from build123d import *

# Parameters (mm, degrees)
SKETCH1_R           = 5
BOSS_EXTRUDE1_DEPTH = 8
SKETCH2_R           = 17.5
BOSS_EXTRUDE2_DEPTH = 5
BOSS_EXTRUDE3_START = 7.75
SKETCH3_R           = 17.5
SKETCH3_R_2         = 13.5
BOSS_EXTRUDE3_DEPTH = 7.75
SKETCH4_R           = 6
BOSS_EXTRUDE4_DEPTH = 58.4
SKETCH7_R           = 7.998050104
SKETCH7_R_2         = 4
CUT_EXTRUDE1_DEPTH  = 30
SKETCH8_R           = 8
SKETCH8_R_2         = 6
BOSS_EXTRUDE6_DEPTH = 9
BOSS_EXTRUDE7_START = 5
BOSS_EXTRUDE7_DEPTH = 5


with BuildPart() as part:
    # Sketch1 → Boss-Extrude1 (new body)
    with BuildSketch(Plane(origin=(0, 0, 0), x_dir=(1, 0, 0), z_dir=(0, 1, 0))):
        with Locations(Location((0, 0, 0), (0, 0, 270))):
            Circle(SKETCH1_R)
    extrude(amount=-BOSS_EXTRUDE1_DEPTH)

    # Sketch2 → Boss-Extrude2 (add)
    with BuildSketch(Plane(origin=(0, 0, 0), x_dir=(1, 0, 0), z_dir=(0, 1, 0))):
        with Locations(Location((0, 0, 0), (0, 0, 270))):
            Circle(SKETCH2_R)
    extrude(amount=BOSS_EXTRUDE2_DEPTH)

    # Sketch3 → Boss-Extrude3 (add)
    with BuildSketch(Plane.XZ.offset(BOSS_EXTRUDE3_START)):
        with Locations(Location((0, 0, 0), (0, 0, 270))):
            Circle(SKETCH3_R)
        with Locations(Location((0, 0, 0), (0, 0, 270))):
            Circle(SKETCH3_R_2, mode=Mode.SUBTRACT)
    extrude(amount=-BOSS_EXTRUDE3_DEPTH)

    # Sketch4 → Boss-Extrude4 (add)
    with BuildSketch(Plane(origin=(0, 5, 0), x_dir=(1, 0, 0), z_dir=(0, 1, 0))):
        with Locations(Location((0, 0, 0), (0, 0, 270))):
            Circle(SKETCH4_R)
    extrude(amount=BOSS_EXTRUDE4_DEPTH)

    # Sketch7 → Cut-Extrude1 (cut)
    with BuildSketch(Plane(origin=(0, 63.4, 0), x_dir=(1, 0, 0), z_dir=(0, 1, 0))):
        Circle(SKETCH7_R)
        with Locations(Location((0, 0, 0), (0, 0, 270))):
            Circle(SKETCH7_R_2, mode=Mode.SUBTRACT)
    extrude(amount=-CUT_EXTRUDE1_DEPTH, mode=Mode.SUBTRACT)

    # Sketch8 → Boss-Extrude6 (add)
    with BuildSketch(Plane(origin=(0, 5, 0), x_dir=(1, 0, 0), z_dir=(0, 1, 0))):
        with Locations(Location((0, 0, 0), (0, 0, 270))):
            Circle(SKETCH8_R)
        with Locations(Location((0, 0, 0), (0, 0, 270))):
            Circle(SKETCH8_R_2, mode=Mode.SUBTRACT)
    extrude(amount=BOSS_EXTRUDE6_DEPTH)

    # Sketch10 → Boss-Extrude7 (add)
    with BuildSketch(Plane(origin=(0, 63.4, 0), x_dir=(1, 0, 0), z_dir=(0, 1, 0)).offset(BOSS_EXTRUDE7_START)):
        with BuildLine():
            Line((-3.25, 2.331844763), (-3.25, -2.331844763))
            ThreePointArc((-3.25, -2.331844763), (-2.828427125, -2.828427125), (-2.331844763, -3.25))
            Line((-2.331844763, -3.25), (2.331844763, -3.25))
            ThreePointArc((2.331844763, -3.25), (2.828427125, -2.828427125), (3.25, -2.331844763))
            Line((3.25, -2.331844763), (3.25, 2.331844763))
            ThreePointArc((3.25, 2.331844763), (2.828427125, 2.828427125), (2.331844763, 3.25))
            Line((2.331844763, 3.25), (-2.331844763, 3.25))
            ThreePointArc((-2.331844763, 3.25), (-2.828427125, 2.828427125), (-3.25, 2.331844763))
        make_face()
    extrude(amount=-BOSS_EXTRUDE7_DEPTH)


solid = part.part
Could you check a few things on this model? Use its own coordinates, in mm. A direction names the side the tool comes from. Give positions to 0.01 mm unless a question says otherwise; leave off trailing zeros. Order: outer loops, then holes, each group sorted by start corner. A loop starts at its lowest first (then second) coordinate and runs counter-clockwise, first axis right, second up. Notation, with made-up numbers: (-28, 70) - (29, 70) arc R19 cw to (29, 102) - close; hole circle Ø3 at (-6.75, 37.25). An arc over 180 degrees is marked (long way). One line per item, written item: value. Start each with the question number.
1. Imagine slicing it at B-B on z = 0. List the corners of the cut face in (x, y) for me, plus the area to 3 significant figures.
2. Thinking about a two-plate mould opening in Z: for faces 4 (the face through (6, 14, -2)), 5 (the face through (1.802, 23.564, 5.723)), 6 (the face through (-13.18, -3.93, 2.93)), which applies, +Z half, -Z half, draft (parallel to the pull), parting line (faces both ways), or undercut?
3. For faces 1 (the face through (0, 66, -3.25)), 2 (the face through (-4.88, -3.94, -1.08)), 3 (the face through (-7.81, 9.44, -1.73)), which set-ups out of +Z, -Z, +X, -X, +Y, -Y let a thin tool reach every point of the face, with its end or its side?
4. For P1, Ø3, axis at x = 14, y = -0.5, coming from the -Z side; P2, Ø0.6, axis at x = 0.5, z = 3.5, coming from the +Y side; P3, Ø3.5, axis at x = 0, y = 65, coming from the -Z side; P4, Ø5, axis at y = 65.5, z = 0, coming from the +X side, each with a flat end and sliding along its axis, tell me the tip position at first contact or that it passes through.
5. If I drill on probe 1 along X at (y, z) = (-1.75, 0); probe 2 along Y at (x, z) = (11.5, -3.5); probe 3 along Y at (x, z) = (-13.5, 10.5), over which ranges is the centre line in solid material (lowest first)?
6. Imagine slicing it at A-A on x = 0. List the corners of the cut face in (y, z) for me.
7. Imagine slicing it at C-C on y = 62. List the corners of the cut face in (x, z) for me.
8. Imagine slicing it at D-D on y = 32.5. List the corners of the cut face in (x, z) for me.
Values:
1. outline: (-17.5, -7.75) - (-13.5, -7.75) - (-13.5, 0) - (-5, 0) - (-5, -8) - (5, -8) - (5, 0) - (13.5, 0) - (13.5, -7.75) - (17.5, -7.75) - (17.5, 5) - (8, 5) - (8, 14) - (6, 14) - (6, 33.4) - (4, 33.4) - (4, 63.4) - (3.25, 63.4) - (3.25, 68.4) - (-3.25, 68.4) - (-3.25, 63.4) - (-4, 63.4) - (-4, 33.4) - (-6, 33.4) - (-6, 14) - (-8, 14) - (-8, 5) - (-17.5, 5) - close
1. area: 966 mm²
2. face 4: draft
2. face 5: parting line
2. face 6: undercut
3. face 1: -Z, +X, -X, +Y
3. face 2: -Y
3. face 3: +Y
4. P1: z = -12.25
4. P2: y = 68.4
4. P3: z = -4
4. P4: x = 4
5. probe 1: -17.5 to -13.5, -5 to 5, 13.5 to 17.5
5. probe 2: 0 to 5
5. probe 3: -7.75 to 5
6. outline: (-8, -5) - (0, -5) - (0, -13.5) - (-7.75, -13.5) - (-7.75, -17.5) - (5, -17.5) - (5, -8) - (14, -8) - (14, -6) - (33.4, -6) - (33.4, -4) - (63.4, -4) - (63.4, -3.25) - (68.4, -3.25) - (68.4, 3.25) - (63.4, 3.25) - (63.4, 4) - (33.4, 4) - (33.4, 6) - (14, 6) - (14, 8) - (5, 8) - (5, 17.5) - (-7.75, 17.5) - (-7.75, 13.5) - (0, 13.5) - (0, 5) - (-8, 5) - close
7. outline: circle Ø8 at (0, 0)
8. outline: circle Ø12 at (0, 0)
